from build123d import *

# Parameters (mm, degrees)
EXTRUSION1_DEPTH = 48
EXTRUSION3_REACH = 32.949
ESQUISSE2_R      = 1.5
ESQUISSE2_W      = 20
ESQUISSE2_H      = 32
CONG_1_R         = 3
EXTRUSION4_REACH = 5
ESQUISSE3_R      = 1.1


with BuildPart() as part:
    # Esquisse1 → Extrusion1 (new body)
    with BuildSketch(Plane(origin=(0, 0, 0), x_dir=(1, 0, 0), z_dir=(0, 1, 0))):
        with BuildLine():
            Line((0, 0), (0, 30))
            Line((0, 30), (3, 30))
            Line((3, 30), (3, 0))
            ThreePointArc((3, 0), (4.257195182, -12.918344113), (7.981600437, -25.351885839))
            Line((7.981600437, -25.351885839), (15.549327553, -43.864840933))
            Line((15.549327553, -43.864840933), (12.772384289, -45))
            Line((12.772384289, -45), (5.204657173, -26.487044906))
            ThreePointArc((5.204657173, -26.487044906), (1.313487503, -13.496777432), (0, 0))
        make_face()
    extrude(amount=EXTRUSION1_DEPTH)

    # Esquisse2 → Extrusion3 (cut, up to next)
    with BuildSketch(Plane(origin=(-4.817679226, 0, 1.969371261), x_dir=(0.378386356, 0, 0.925647755), z_dir=(-0.925647755, 0, 0.378386356)), mode=Mode.PRIVATE) as extrusion3_sk1:
        with Locations((42.487044906, 4)):
            Circle(ESQUISSE2_R)
    extrusion3_tool1 = extrude(extrusion3_sk1.sketch, amount=-EXTRUSION3_REACH, mode=Mode.PRIVATE) & part.part
    add(extrusion3_tool1.solids().sort_by_distance((11.258839, 4, 41.297409))[0], mode=Mode.SUBTRACT)
    # Esquisse2 → Extrusion3 (cut, up to next)
    with BuildSketch(Plane(origin=(-4.817679226, 0, 1.969371261), x_dir=(0.378386356, 0, 0.925647755), z_dir=(-0.925647755, 0, 0.378386356)), mode=Mode.PRIVATE) as extrusion3_sk2:
        with Locations((42.487044906, 44)):
            Circle(ESQUISSE2_R)
    extrusion3_tool2 = extrude(extrusion3_sk2.sketch, amount=-EXTRUSION3_REACH, mode=Mode.PRIVATE) & part.part
    add(extrusion3_tool2.solids().sort_by_distance((11.258839, 44, 41.297409))[0], mode=Mode.SUBTRACT)
    # Esquisse2 → Extrusion3 (cut, up to next)
    with BuildSketch(Plane(origin=(-4.817679226, 0, 1.969371261), x_dir=(0.378386356, 0, 0.925647755), z_dir=(-0.925647755, 0, 0.378386356)), mode=Mode.PRIVATE) as extrusion3_sk3:
        with Locations((36.487044906, 24)):
            Rectangle(ESQUISSE2_W, ESQUISSE2_H)
    extrusion3_tool3 = extrude(extrusion3_sk3.sketch, amount=-EXTRUSION3_REACH, mode=Mode.PRIVATE) & part.part
    add(extrusion3_tool3.solids().sort_by_distance((8.988521, 24, 35.743522))[0], mode=Mode.SUBTRACT)

    # Congé1
    cong_1_edges = [part.edges().sort_by_distance(p)[0] for p in [
        (14.160855921, 48, 44.432420466),
        (14.160855921, 0, 44.432420466),
    ]]
    fillet(cong_1_edges, radius=CONG_1_R)

    # Esquisse3 → Extrusion4 (cut, up to next)
    with BuildSketch(Plane(origin=(3, 0, 0), x_dir=(0, 0, -1), z_dir=(1, 0, 0)), mode=Mode.PRIVATE) as extrusion4_sk1:
        with Locations((3, 16)):
            Circle(ESQUISSE3_R)
    extrusion4_tool1 = extrude(extrusion4_sk1.sketch, amount=-EXTRUSION4_REACH, mode=Mode.PRIVATE) & part.part
    add(extrusion4_tool1.solids().sort_by_distance((3, 16, -3))[0], mode=Mode.SUBTRACT)
    # Esquisse3 → Extrusion4 (cut, up to next)
    with BuildSketch(Plane(origin=(3, 0, 0), x_dir=(0, 0, -1), z_dir=(1, 0, 0)), mode=Mode.PRIVATE) as extrusion4_sk2:
        with Locations((11, 16)):
            Circle(ESQUISSE3_R)
    extrusion4_tool2 = extrude(extrusion4_sk2.sketch, amount=-EXTRUSION4_REACH, mode=Mode.PRIVATE) & part.part
    add(extrusion4_tool2.solids().sort_by_distance((3, 16, -11))[0], mode=Mode.SUBTRACT)
    # Esquisse3 → Extrusion4 (cut, up to next)
    with BuildSketch(Plane(origin=(3, 0, 0), x_dir=(0, 0, -1), z_dir=(1, 0, 0)), mode=Mode.PRIVATE) as extrusion4_sk3:
        with Locations((19, 16)):
            Circle(ESQUISSE3_R)
    extrusion4_tool3 = extrude(extrusion4_sk3.sketch, amount=-EXTRUSION4_REACH, mode=Mode.PRIVATE) & part.part
    add(extrusion4_tool3.solids().sort_by_distance((3, 16, -19))[0], mode=Mode.SUBTRACT)
    # Esquisse3 → Extrusion4 (cut, up to next)
    with BuildSketch(Plane(origin=(3, 0, 0), x_dir=(0, 0, -1), z_dir=(1, 0, 0)), mode=Mode.PRIVATE) as extrusion4_sk4:
        with Locations((3, 24)):
            Circle(ESQUISSE3_R)
    extrusion4_tool4 = extrude(extrusion4_sk4.sketch, amount=-EXTRUSION4_REACH, mode=Mode.PRIVATE) & part.part
    add(extrusion4_tool4.solids().sort_by_distance((3, 24, -3))[0], mode=Mode.SUBTRACT)
    # Esquisse3 → Extrusion4 (cut, up to next)
    with BuildSketch(Plane(origin=(3, 0, 0), x_dir=(0, 0, -1), z_dir=(1, 0, 0)), mode=Mode.PRIVATE) as extrusion4_sk5:
        with Locations((19, 24)):
            Circle(ESQUISSE3_R)
    extrusion4_tool5 = extrude(extrusion4_sk5.sketch, amount=-EXTRUSION4_REACH, mode=Mode.PRIVATE) & part.part
    add(extrusion4_tool5.solids().sort_by_distance((3, 24, -19))[0], mode=Mode.SUBTRACT)
    # Esquisse3 → Extrusion4 (cut, up to next)
    with BuildSketch(Plane(origin=(3, 0, 0), x_dir=(0, 0, -1), z_dir=(1, 0, 0)), mode=Mode.PRIVATE) as extrusion4_sk6:
        with Locations((19, 32)):
            Circle(ESQUISSE3_R)
    extrusion4_tool6 = extrude(extrusion4_sk6.sketch, amount=-EXTRUSION4_REACH, mode=Mode.PRIVATE) & part.part
    add(extrusion4_tool6.solids().sort_by_distance((3, 32, -19))[0], mode=Mode.SUBTRACT)
    # Esquisse3 → Extrusion4 (cut, up to next)
    with BuildSketch(Plane(origin=(3, 0, 0), x_dir=(0, 0, -1), z_dir=(1, 0, 0)), mode=Mode.PRIVATE) as extrusion4_sk7:
        with Locations((11, 32)):
            Circle(ESQUISSE3_R)
    extrusion4_tool7 = extrude(extrusion4_sk7.sketch, amount=-EXTRUSION4_REACH, mode=Mode.PRIVATE) & part.part
    add(extrusion4_tool7.solids().sort_by_distance((3, 32, -11))[0], mode=Mode.SUBTRACT)
    # Esquisse3 → Extrusion4 (cut, up to next)
    with BuildSketch(Plane(origin=(3, 0, 0), x_dir=(0, 0, -1), z_dir=(1, 0, 0)), mode=Mode.PRIVATE) as extrusion4_sk8:
        with Locations((3, 32)):
            Circle(ESQUISSE3_R)
    extrusion4_tool8 = extrude(extrusion4_sk8.sketch, amount=-EXTRUSION4_REACH, mode=Mode.PRIVATE) & part.part
    add(extrusion4_tool8.solids().sort_by_distance((3, 32, -3))[0], mode=Mode.SUBTRACT)


solid = part.part
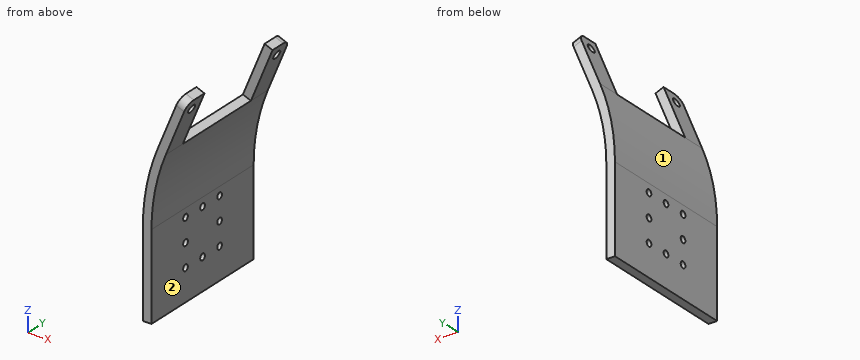
Could you check a few things on this model? Use its own coordinates, in mm. Face numbers are marked on the shaded views. A direction names the side the tool comes from. Round coordinates to 2 decimals unless told otherwise and drop trailing zeros. Order: outer loops, then holes, each group sorted by start corner. A loop starts at its lowest first (then second) coordinate and runs counter-clockwise, first axis right, second up.
(1) Imagine slicing it at C-C (z = -3). Write out the boundary of the cut face in (x, y), plus the area to 3 significant figures.
Response values:
outline: (0, 0) - (3, 0) - (3, 14.9) - (0, 14.9) - close; (0, 17.1) - (3, 17.1) - (3, 22.9) - (0, 22.9) - close; (0, 25.1) - (3, 25.1) - (3, 30.9) - (0, 30.9) - close; (0, 33.1) - (3, 33.1) - (3, 48) - (0, 48) - close
area: 124 mm2
(2) I'm going to push flat-ended pins straight in: pin 1 (1.3 mm diameter, centred on y = 16, z = -11, fed in from +X); pin 2 (1 mm diameter, centred on x = 11.5, y = 42.5, fed in from -Z); pin 3 (3 mm diameter, centred on y = 32, z = -11, fed in from +X); pin 4 (2 mm diameter, centred on y = 7, z = 29.5, fed in from +X). Where does each tip first touch, or does it pass through?
Response values:
pin 1: passes through
pin 2: stops at z = 32.74
pin 3: stops at x = 3
pin 4: stops at x = 10.09
(3) Imagine slicing it at D-D (x = 9). Write out the boundary of the cut face in (y, z), plus the area to 3 significant figures.
Response values:
outline: (0, 27.84) - (8, 27.84) - (8, 35.77) - (0, 35.77) - close; (40, 27.84) - (48, 27.84) - (48, 35.77) - (40, 35.77) - close
area: 127 mm2
(4) Imagine slicing it at A-A (z = -11). Write out the boundary of the cut face in (x, y).
Response values:
outline: (0, 0) - (3, 0) - (3, 14.9) - (0, 14.9) - close; (0, 17.1) - (3, 17.1) - (3, 30.9) - (0, 30.9) - close; (0, 33.1) - (3, 33.1) - (3, 48) - (0, 48) - close
(5) Imagine slicing it at B-B (y = 24). Write out the boundary of the cut face in (x, z), plus the area to 3 significant figures.
Response values:
outline: (0, -30) - (3, -30) - (3, -20.1) - (0, -20.1) - close; (0, -17.9) - (3, -17.9) - (3, -4.1) - (0, -4.1) - close; (0, -1.9) - (3, -1.9) - (3, 0) arc R67 cw to (7.98, 25.35) - (5.2, 26.49) arc R70 ccw to (0, 0) - close
area: 157 mm2
(6) Please list where these lines run through material, in increasing order: line 1 along Y through (x, z) = (1.6, -19); line 2 along Y through (x, z) = (0.8, -11); line 3 along Y through (x, z) = (10.5, 34).
Response values:
line 1: y = 0 to 14.9, 17.1 to 22.9, 25.1 to 30.9, 33.1 to 48
line 2: y = 0 to 14.9, 17.1 to 30.9, 33.1 to 48
line 3: y = 0 to 8, 40 to 48
(7) Which directions (+Z, -Z, +X, -X, +Y, -Y) give clear straight access to the entire face, cutting with the end or side of a thin tool? Please do the marked faces 1 and 2.
Response values:
face 1: +Z, -X, +Y, -Y
face 2: -Z, +X, +Y, -Y
